from build123d import *

# Parameters (mm, degrees)
SKETCH_1_W          = 100
SKETCH_1_H          = 72
EXTRUDE_1_DEPTH     = 5
SKETCH_1_H_2        = 23
EXTRUDE_1_2_DEPTH   = 5
SKETCH_1_3_W        = 100
SKETCH_1_3_H        = 5
EXTRUDE_2_DEPTH     = 30
SKETCH_2_W          = 100
SKETCH_2_H          = 5
EXTRUDE_3_DEPTH     = 23
SKETCH_3_R          = 2.1
CUT_EXTRUDE_1_DEPTH = 77.811457479
FILLET_1_R          = 3
EXTRUDE_4_DEPTH     = 100


with BuildPart() as part:
    # Sketch 1 → Extrude 1 (new body)
    with BuildSketch(Plane.XY):
        with Locations((0, -14)):
            Rectangle(SKETCH_1_W, SKETCH_1_H)
    extrude(amount=EXTRUDE_1_DEPTH)



with BuildPart() as body_2:
    # Sketch 1 → Extrude 1 2 (new body)
    with BuildSketch(Plane.XY):
        with Locations((0, 38.5)):
            Rectangle(SKETCH_1_W, SKETCH_1_H_2)
    extrude(amount=EXTRUDE_1_2_DEPTH)


with BuildPart() as part_1:
    add(part.part)

    add(body_2.part)  # Extrude 2 merges body 2
    # Sketch 1_3 → Extrude 2 (add)
    with BuildSketch(Plane.XY):
        with Locations((0, 24.5)):
            Rectangle(SKETCH_1_3_W, SKETCH_1_3_H)
    extrude(amount=EXTRUDE_2_DEPTH)

    # Sketch 2 → Extrude 3 (add)
    with BuildSketch(Plane(origin=(0, 27, 0), x_dir=(1, 0, 0), z_dir=(0, 1, 0))):
        with Locations((0, -27.5)):
            Rectangle(SKETCH_2_W, SKETCH_2_H)
    extrude(amount=EXTRUDE_3_DEPTH)

    # Sketch 3 → Cut-Extrude 1 (cut, through all)
    with BuildSketch(Plane.XY.offset(30)):
        with Locations((-40, 40)):
            Circle(SKETCH_3_R)
        with Locations((0, 40)):
            Circle(SKETCH_3_R)
        with Locations((40, 40)):
            Circle(SKETCH_3_R)
    extrude(amount=-CUT_EXTRUDE_1_DEPTH, mode=Mode.SUBTRACT)

    # Fillet 1
    fillet_1_edges = [part_1.edges().sort_by_distance(p)[0] for p in [
        (0, 27, 5),
        (0, 27, 25),
    ]]
    fillet(fillet_1_edges, radius=FILLET_1_R)

    # Sketch 8 → Extrude 4 (add, through all)
    with BuildSketch(Plane.ZY.offset(50)):
        Polygon((5, 19), (8, 22), (5, 22), align=None)
    extrude(amount=-EXTRUDE_4_DEPTH)


solid = part_1.part
Could you check a few things on this model? Use its own coordinates, in mm. A direction names the side the tool comes from. Coordinates: 2 decimals unless noted, no trailing zeros. Order: outer loops, then holes, each group sorted by start corner. A loop starts at its lowest first (then second) coordinate and runs counter-clockwise, first axis right, second up. Notation, with made-up numbers: (-31, 82) -> (7, 82) arc R19 cw to (7, 100) -> close; hole circle Ø7 at (72, 1.25). An arc over 180 degrees is marked (long way). One line per item, written item: value. Start each with the question number.
1) Imagine slicing it at D-D on x = 11. List the corners of the cut face in (y, z) for me.
2) If I drill on L1, parallel to Y at x = 40, z = 3.6; L2, parallel to Y at x = -40, z = 27.6; L3, parallel to Z at x = 14, y = -41.5, over which ranges is the centre line in solid material (lowest first)? Write a range as [from, to].
3) Imagine slicing it at B-B on x = -40. List the corners of the cut face in (y, z) for me, plus the area to 3 significant figures.
4) Imagine slicing it at C-C on y = 40. Count the separate pieces of the cut face and the enclosed holes in it, plus the area to 3 significant figures.
5) I'm going to push flat-ended pins straight in: pin 1 (5.5 mm diameter, centred on x = 0, y = 40, fed in from -Z); pin 2 (4 mm diameter, centred on x = 21, z = 11, fed in from -Y); pin 3 (1.5 mm diameter, centred on x = -16.5, z = 7, fed in from +Y); pin 4 (11 mm diameter, centred on x = -10.5, z = 17.5, fed in from +Y). Where does each tip first touch, or does it pass through?
6) Which directions (+Z, -Z, +X, -X, +Y, -Y) give clear straight access to the entire face, cutting with the end or side of a thin tool? Please do faces 5 (the flat face through (-1, 22, 19)), 6 (the cylindrical face through (0.7, 27.86, 5.9)), 7 (the cylindrical face through (38.334, 38.722, 2.535)).
7) We'd pull the mould along X, two halves only. Please class faces 1 (the flat face through (-50, 11, 4)), 2 (the cylindrical face through (-0.46, 37.95, 2.54)), 3 (the flat face through (-1, 27, 15)), 4 (the cylindrical face through (-41.666, 38.722, 27.535)): +X half, -X half, draft (parallel to the pull), parting line (faces both ways), or undercut.
8) Imagine slicing it at A-A on z = 26.5. List the corners of the cut face in (x, y) for me, plus the area to 3 significant figures.
Answer list:
1. outline: (-50, 0) -> (50, 0) -> (50, 5) -> (30, 5) arc R3 cw to (27, 8) -> (27, 22) arc R3 cw to (30, 25) -> (50, 25) -> (50, 30) -> (22, 30) -> (22, 8) -> (19, 5) -> (-50, 5) -> close
2. L1: y = [-50, 37.9], [42.1, 50]
2. L2: y = [22, 37.9], [42.1, 50]
2. L3: z = [0, 5]
3. outline: (-50, 0) -> (37.9, 0) -> (37.9, 5) -> (30, 5) arc R3 cw to (27, 8) -> (27, 22) arc R3 cw to (30, 25) -> (37.9, 25) -> (37.9, 30) -> (22, 30) -> (22, 8) -> (19, 5) -> (-50, 5) -> close; (42.1, 0) -> (50, 0) -> (50, 5) -> (42.1, 5) -> close; (42.1, 25) -> (50, 25) -> (50, 30) -> (42.1, 30) -> close
3. area: 706 mm2
4. separate pieces: 8
4. enclosed holes: 0
4. area: 874 mm2
5. pin 1: stops at z = 0
5. pin 2: stops at y = 22
5. pin 3: stops at y = 27.56
5. pin 4: stops at y = 27.17
6. face 5: +Z, +X, -X, -Y
6. face 6: +X, -X, +Y
6. face 7: +Z, -Z
7. face 1: -X half
7. face 2: undercut
7. face 3: draft
7. face 4: undercut
8. outline: (-50, 22) -> (50, 22) -> (50, 50) -> (-50, 50) -> close; hole circle Ø4.2 at (-40, 40); hole circle Ø4.2 at (0, 40); hole circle Ø4.2 at (40, 40)
8. area: 2,760 mm2
